Here's how the part is built. I have some questions about the finished solid (model axes, mm). A direction names the side the tool comes from. Round coordinates to 2 decimals unless told otherwise and drop trailing zeros. Order: outer loops, then holes, each group sorted by start corner. A loop starts at its lowest first (then second) coordinate and runs counter-clockwise, first axis right, second up.
```python
from build123d import *

# Parameters (mm, degrees)
PAD_DEPTH       = 5
SKETCH001_W     = 36.2
SKETCH001_H     = 26.2
POCKET_DEPTH    = 4.5
SKETCH002_W     = 14.7
SKETCH002_H     = 10.7
POCKET001_DEPTH = 4
SKETCH003_R     = 1.25
PAD001_DEPTH    = 4
SKETCH004_R     = 0.5
POCKET002_DEPTH = 1.001
SKETCH005_R     = 1.75
POCKET003_DEPTH = 5.001
POCKET004_DEPTH = 2.5
SKETCH007_W     = 4.7
SKETCH007_H     = 4.7
POCKET005_DEPTH = 3.7
SKETCH008_W     = 6
SKETCH008_H     = 4.5
POCKET006_DEPTH = 2.3
SKETCH009_W     = 0.6
SKETCH009_H     = 5.8
POCKET007_DEPTH = 2.3
SKETCH010_W     = 2.8
SKETCH010_H     = 7.6
POCKET008_DEPTH = 2.8
SKETCH011_W     = 0.6
SKETCH011_H     = 3.5
POCKET009_DEPTH = 2.3
SKETCH012_R     = 6
POCKET010_DEPTH = 4.5
POCKET011_DEPTH = 4.5
SKETCH014_W     = 2.15
SKETCH014_H     = 0.8
POCKET012_DEPTH = 2.3
POCKET013_DEPTH = 0.6
POCKET014_DEPTH = 1
SKETCH017_R     = 0.25
POCKET015_DEPTH = 0.501


with BuildPart() as part:
    # Sketch → Pad (new body)
    with BuildSketch(Plane.XY):
        Polygon((-25, 14.433757), (-25, -14.433757), (0, -28.867513), (25, -14.433757), (25, 14.433757), (0, 28.867513), align=None)
    extrude(amount=PAD_DEPTH)

    # Sketch001 → Pocket (cut)
    with BuildSketch(Plane.XY.offset(5)):
        with Locations((-5.9, -0.9)):
            Rectangle(SKETCH001_W, SKETCH001_H)
    extrude(amount=-POCKET_DEPTH, mode=Mode.SUBTRACT)

    # Sketch002 → Pocket001 (cut)
    with BuildSketch(Plane.XY.offset(5)):
        with Locations((0, 18.55)):
            Rectangle(SKETCH002_W, SKETCH002_H)
    extrude(amount=-POCKET001_DEPTH, mode=Mode.SUBTRACT)

    # Sketch003 → Pad001 (new body)
    with BuildSketch(Plane.XY.offset(1)):
        with Locations((-4.45, 21.2)):
            Circle(SKETCH003_R)
    extrude(amount=PAD001_DEPTH)

    # Sketch004 → Pocket002 (cut, through all)
    with BuildSketch(Plane.XY.offset(1)):
        with Locations((-3.5, 15.3)):
            Circle(SKETCH004_R)
    extrude(amount=-POCKET002_DEPTH, mode=Mode.SUBTRACT)

    # Sketch005 → Pocket003 (cut, through all)
    with BuildSketch(Plane.XY.offset(5)):
        with Locations((10.75, 18.619546)):
            Circle(SKETCH005_R)
        with Locations((-10.75, -18.619546)):
            Circle(SKETCH005_R)
    extrude(amount=-POCKET003_DEPTH, mode=Mode.SUBTRACT)

    # Sketch006 → Pocket004 (cut)
    with BuildSketch(Plane(origin=(0, 0, 0), x_dir=(1, 0, 0), z_dir=(0, 0, -1))):
        Polygon((-13.05, 17.291641), (-10.75, 15.963735), (-8.45, 17.291641), (-8.45, 19.947452), (-10.75, 21.275357), (-13.05, 19.947452), align=None)
        Polygon((10.75, -21.275357), (13.05, -19.947452), (13.05, -17.291641), (10.75, -15.963735), (8.45, -17.291641), (8.45, -19.947452), align=None)
    extrude(amount=-POCKET004_DEPTH, mode=Mode.SUBTRACT)

    # Sketch007 → Pocket005 (cut)
    with BuildSketch(Plane.XY.offset(5)):
        with Locations((17.35, -11.65)):
            Rectangle(SKETCH007_W, SKETCH007_H)
    extrude(amount=-POCKET005_DEPTH, mode=Mode.SUBTRACT)

    # Sketch008 → Pocket006 (cut)
    with BuildSketch(Plane.XY.offset(5)):
        with Locations((17.35, -7.05)):
            Rectangle(SKETCH008_W, SKETCH008_H)
    extrude(amount=-POCKET006_DEPTH, mode=Mode.SUBTRACT)

    # Sketch009 → Pocket007 (cut)
    with BuildSketch(Plane.XY.offset(5)):
        with Locations((17.35, -1.9)):
            Rectangle(SKETCH009_W, SKETCH009_H)
    extrude(amount=-POCKET007_DEPTH, mode=Mode.SUBTRACT)

    # Sketch010 → Pocket008 (cut)
    with BuildSketch(Plane.XY.offset(5)):
        with Locations((17.35, 4.8)):
            Rectangle(SKETCH010_W, SKETCH010_H)
    extrude(amount=-POCKET008_DEPTH, mode=Mode.SUBTRACT)

    # Sketch011 → Pocket009 (cut)
    with BuildSketch(Plane.XY.offset(5)):
        with Locations((17.35, 10.35)):
            Rectangle(SKETCH011_W, SKETCH011_H)
    extrude(amount=-POCKET009_DEPTH, mode=Mode.SUBTRACT)

    # Sketch012 → Pocket010 (cut)
    with BuildSketch(Plane.XY.offset(5)):
        with Locations((0, -21)):
            Circle(SKETCH012_R)
    extrude(amount=-POCKET010_DEPTH, mode=Mode.SUBTRACT)

    # Sketch013 → Pocket011 (cut)
    with BuildSketch(Plane.XY.offset(5)):
        Polygon((-0.841162, -17.860741), (6.403282, -15.919598), (8.085606, -22.198116), (0.841162, -24.139259), align=None)
    extrude(amount=-POCKET011_DEPTH, mode=Mode.SUBTRACT)

    # Sketch014 → Pocket012 (cut)
    with BuildSketch(Plane.XY.offset(5)):
        with Locations((13.275, -7.05)):
            Rectangle(SKETCH014_W, SKETCH014_H)
    extrude(amount=-POCKET012_DEPTH, mode=Mode.SUBTRACT)

    # Sketch015 → Pocket013 (cut)
    with BuildSketch(Plane.XY.offset(5)):
        Polygon((21.1, 3.15), (24.7, 3.15), (24.7, 2), (25.4, 2), (25.4, -2), (24.7, -2), (24.7, -3.15), (21.1, -3.15), align=None)
    extrude(amount=-POCKET013_DEPTH, mode=Mode.SUBTRACT)

    # Sketch016 → Pocket014 (cut)
    with BuildSketch(Plane.XY.offset(5)):
        Polygon((20.35, -5.8), (21.1, -5.8), (21.1, -3.15), (21.7, -3.15), (21.7, -6.4), (20.35, -6.4), align=None)
    extrude(amount=-POCKET014_DEPTH, mode=Mode.SUBTRACT)

    # Sketch017 → Pocket015 (cut, through all)
    with BuildSketch(Plane.XY.offset(0.5)):
        Circle(SKETCH017_R)
    extrude(amount=-POCKET015_DEPTH, mode=Mode.SUBTRACT)


solid = part.part
```
1. If we section it at A-A, the plane y = 11: Write out the boundary of the cut face in (x, z).
Evaluation:
outline: (-25, 0) - (25, 0) - (25, 5) - (17.65, 5) - (17.65, 2.7) - (17.05, 2.7) - (17.05, 5) - (12.2, 5) - (12.2, 0.5) - (-24, 0.5) - (-24, 5) - (-25, 5) - close
2. If we section it at C-C, the plane x = 5: Write out the boundary of the cut face in (y, z).
Evaluation:
outline: (-25.98, 0) - (25.98, 0) - (25.98, 5) - (23.9, 5) - (23.9, 1) - (13.2, 1) - (13.2, 5) - (12.2, 5) - (12.2, 0.5) - (-14, 0.5) - (-14, 5) - (-16.3, 5) - (-16.3, 0.5) - (-24.32, 0.5) - (-24.32, 5) - (-25.98, 5) - close
3. On a 3-axis mill with a long thin cutter (end or side, diameter ignored), from which of +Z, -Z, +X, -X, +Y, -Y can I reach the whole of each face in a straight line? I mean faces 1 (the cylindrical face through (-9.94, -20.17, 3.77)), 2 (the flat face through (17, -14, 3)), 3 (the flat face through (9.58, 20.6, 1.23)). Say none if no direction works.
Evaluation:
face 1: +Z, -Z
face 2: +Z
face 3: -Z
4. If we section it at B-B, the plane x = -18: Write out the boundary of the cut face in (y, z).
Evaluation:
outline: (-18.48, 0) - (18.48, 0) - (18.48, 5) - (12.2, 5) - (12.2, 0.5) - (-14, 0.5) - (-14, 5) - (-18.48, 5) - close
5. I need wall thicknesses on probe 1 along Y at (x, z) = (0, 4); probe 2 along X at (y, z) = (-21, 1.65); probe 3 along Y at (x, z) = (-4, 3.9). Which ranges of each line are inside material? Lowest first, please.
Evaluation:
probe 1: y = -28.87 to -27, -15 to -14, 12.2 to 13.2, 23.9 to 28.87
probe 2: x = -13.63 to -11.23, -10.27 to -6, 7.76 to 13.63
probe 3: y = -26.56 to -25.47, -16.53 to -14, 12.2 to 13.2, 20.03 to 22.37, 23.9 to 26.56
6. I'm going to push flat-ended pins straight in: P1, Ø2, axis at y = -19, z = 1, coming from the -X side; P2, Ø3, axis at x = -2, z = 3.5, coming from the +Y side; P3, Ø0.8, axis at x = 17, y = 4, coming from the +Z side; P4, Ø2, axis at x = -10.75, y = -18.62, coming from the +Z side. Where does each tip first touch, or does it pass through?
Evaluation:
P1: stops at x = -18.82
P2: stops at y = 28.58
P3: stops at z = 2.2
P4: passes through
7. If we mould it in two halves opening along Y, with no side actions, what happens to faces 4 (the flat face through (-13.05, -19, 1)), 5 (the flat face through (15, -12, 3)), 6 (the flat face through (-4, 21, 5))? For each: released by +Y, released by -Y, zero draft, split by the parting line, or undercut.
Evaluation:
face 4: undercut
face 5: undercut
face 6: zero draft
